from build123d import *

# Parameters (mm, degrees)
PAD_DEPTH       = 27
SKETCH001_R     = 16.5
POCKET_DEPTH    = 25
SKETCH002_R     = 16.5
POCKET001_DEPTH = 25
SKETCH003_R     = 16.5
POCKET002_DEPTH = 25
SKETCH004_R     = 16.5
POCKET003_DEPTH = 25
SKETCH005_R     = 16.5
POCKET004_DEPTH = 25
SKETCH006_R     = 16.5
POCKET005_DEPTH = 25
SKETCH007_R     = 5.125
POCKET006_DEPTH = 1.15
SKETCH008_R     = 5.125
POCKET007_DEPTH = 1.15
SKETCH009_W     = 20
SKETCH009_H     = 20
POCKET008_DEPTH = 25


with BuildPart() as part:
    # Sketch → Pad (new body)
    with BuildSketch(Plane.XY):
        with BuildLine():
            ThreePointArc((71.830952, -16.5), (78.374369, 12.374369), (49.5, 5.830952))
            ThreePointArc((49.5, 5.830952), (33, 17.5), (16.5, 5.830952))
            ThreePointArc((16.5, 5.830952), (-12.374369, 12.374369), (-5.830952, -16.5))
            ThreePointArc((-5.830952, -16.5), (-12.374369, -45.374369), (16.5, -38.830952))
            ThreePointArc((16.5, -38.830952), (33, -50.5), (49.5, -38.830952))
            ThreePointArc((49.5, -38.830952), (78.374369, -45.374369), (71.830952, -16.5))
        make_face()
        with BuildLine():
            ThreePointArc((5.830952, -16.5), (7.543698, -15.790586), (9.171788, -14.903969))
            ThreePointArc((9.171788, -14.903969), (9, -16.5), (9.171788, -18.096031))
            ThreePointArc((9.171788, -18.096031), (7.543698, -17.209414), (5.830952, -16.5))
        make_face(mode=Mode.SUBTRACT)
        with BuildLine():
            ThreePointArc((47.903969, -9.171788), (48.790586, -7.543698), (49.5, -5.830952))
            ThreePointArc((49.5, -5.830952), (50.209414, -7.543698), (51.096031, -9.171788))
            ThreePointArc((51.096031, -9.171788), (49.5, -9), (47.903969, -9.171788))
        make_face(mode=Mode.SUBTRACT)
        with BuildLine():
            ThreePointArc((18.096031, -23.828212), (17.209414, -25.456302), (16.5, -27.169048))
            ThreePointArc((16.5, -27.169048), (15.790586, -25.456302), (14.903969, -23.828212))
            ThreePointArc((14.903969, -23.828212), (16.5, -24), (18.096031, -23.828212))
        make_face(mode=Mode.SUBTRACT)
        with BuildLine():
            ThreePointArc((47.903969, -23.828212), (49.5, -24), (51.096031, -23.828212))
            ThreePointArc((51.096031, -23.828212), (50.209414, -25.456302), (49.5, -27.169048))
            ThreePointArc((49.5, -27.169048), (48.790586, -25.456302), (47.903969, -23.828212))
        make_face(mode=Mode.SUBTRACT)
        with BuildLine():
            ThreePointArc((14.903969, -9.171788), (15.790586, -7.543698), (16.5, -5.830952))
            ThreePointArc((16.5, -5.830952), (17.209414, -7.543698), (18.096031, -9.171788))
            ThreePointArc((18.096031, -9.171788), (16.5, -9), (14.903969, -9.171788))
        make_face(mode=Mode.SUBTRACT)
        with BuildLine():
            ThreePointArc((23.828212, -18.096031), (24, -16.5), (23.828212, -14.903969))
            ThreePointArc((23.828212, -14.903969), (25.456302, -15.790586), (27.169048, -16.5))
            ThreePointArc((27.169048, -16.5), (25.456302, -17.209414), (23.828212, -18.096031))
        make_face(mode=Mode.SUBTRACT)
        with BuildLine():
            ThreePointArc((42.171788, -18.096031), (40.543698, -17.209414), (38.830952, -16.5))
            ThreePointArc((38.830952, -16.5), (40.543698, -15.790586), (42.171788, -14.903969))
            ThreePointArc((42.171788, -14.903969), (42, -16.5), (42.171788, -18.096031))
        make_face(mode=Mode.SUBTRACT)
        with BuildLine():
            ThreePointArc((56.828212, -18.096031), (57, -16.5), (56.828212, -14.903969))
            ThreePointArc((56.828212, -14.903969), (58.456302, -15.790586), (60.169048, -16.5))
            ThreePointArc((60.169048, -16.5), (58.456302, -17.209414), (56.828212, -18.096031))
        make_face(mode=Mode.SUBTRACT)
    extrude(amount=PAD_DEPTH)

    # Sketch001 (on Face32 of Pad) → Pocket (cut)
    with BuildSketch(Plane.XY.offset(27)):
        Circle(SKETCH001_R)
    extrude(amount=-POCKET_DEPTH, mode=Mode.SUBTRACT)

    # Sketch002 (on Face5 of Pocket) → Pocket001 (cut)
    with BuildSketch(Plane.XY.offset(27)):
        with Locations((33, 0)):
            Circle(SKETCH002_R)
    extrude(amount=-POCKET001_DEPTH, mode=Mode.SUBTRACT)

    # Sketch003 (on Face5 of Pocket001) → Pocket002 (cut)
    with BuildSketch(Plane.XY.offset(27)):
        with Locations((66, 0)):
            Circle(SKETCH003_R)
    extrude(amount=-POCKET002_DEPTH, mode=Mode.SUBTRACT)

    # Sketch004 (on Face5 of Pocket002) → Pocket003 (cut)
    with BuildSketch(Plane.XY.offset(27)):
        with Locations((0, -33)):
            Circle(SKETCH004_R)
    extrude(amount=-POCKET003_DEPTH, mode=Mode.SUBTRACT)

    # Sketch005 (on Face5 of Pocket003) → Pocket004 (cut)
    with BuildSketch(Plane.XY.offset(27)):
        with Locations((33, -33)):
            Circle(SKETCH005_R)
    extrude(amount=-POCKET004_DEPTH, mode=Mode.SUBTRACT)

    # Sketch006 (on Face5 of Pocket004) → Pocket005 (cut)
    with BuildSketch(Plane.XY.offset(27)):
        with Locations((66, -33)):
            Circle(SKETCH006_R)
    extrude(amount=-POCKET005_DEPTH, mode=Mode.SUBTRACT)

    # Sketch007 (on Face4 of Pocket005) → Pocket006 (cut)
    with BuildSketch(Plane(origin=(0, 0, 0), x_dir=(1, 0, 0), z_dir=(0, 0, -1))):
        with Locations((16.5, 16.5)):
            Circle(SKETCH007_R)
    extrude(amount=-POCKET006_DEPTH, mode=Mode.SUBTRACT)

    # Sketch008 (on Face4 of Pocket006) → Pocket007 (cut)
    with BuildSketch(Plane(origin=(0, 0, 0), x_dir=(1, 0, 0), z_dir=(0, 0, -1))):
        with Locations((49.5, 16.5)):
            Circle(SKETCH008_R)
    extrude(amount=-POCKET007_DEPTH, mode=Mode.SUBTRACT)

    # Sketch009 (on Face43 of Pocket007) → Pocket008 (cut)
    with BuildSketch(Plane.XY.offset(27)):
        with Locations((0, 10)):
            Rectangle(SKETCH009_W, SKETCH009_H)
        with Locations((33, 10)):
            Rectangle(SKETCH009_W, SKETCH009_H)
        with Locations((66, 10)):
            Rectangle(SKETCH009_W, SKETCH009_H)
        with Locations((0, -45)):
            Rectangle(SKETCH009_W, SKETCH009_H)
        with Locations((33, -45)):
            Rectangle(SKETCH009_W, SKETCH009_H)
        with Locations((66, -45)):
            Rectangle(SKETCH009_W, SKETCH009_H)
    extrude(amount=-POCKET008_DEPTH, mode=Mode.SUBTRACT)


solid = part.part
Input: part model. Units: mm. Frame: model coordinates. A direction names the side the tool comes from. Give positions to 0.01 mm unless a question says otherwise; leave off trailing zeros. Order: outer loops, then holes, each group sorted by start corner. A loop starts at its lowest first (then second) coordinate and runs counter-clockwise, first axis right, second up. Notation, with made-up numbers: (15.25, -17) -> (53.25, -17) arc R23 cw to (53.25, 21) -> close; hole circle Ø3 at (-1, 73.25). An arc over 180 degrees is marked (long way). Use one line per item in the form item = value.
1) Mould query, pull axis Y, two halves, no side actions, for faces 4 (the cylindrical face through (58.48, -17.2, 13.31)), 5 (the flat face through (18, 8, 27)). Classes: pulls with the +Y half, pulls with the -Y half, needs draft (parallel to the pull), parting line crosses it, or undercut.
Response values:
face_4 = undercut
face_5 = needs draft
2) Line query: probe 1 along X at (y, z) = (4, 18.5); probe 2 along X at (y, z) = (-23.5, 16); probe 3 along Y at (x, z) = (77, 6.5). Output: solid intervals per line, ascending.
Response values:
probe_1 = -17.04 to -16.01, 16.01 to 16.99, 49.01 to 49.99, 82.01 to 83.04
probe_2 = -14.7 to -13.49, 13.49 to 19.51, 46.49 to 52.51, 79.49 to 80.7
probe_3 = -46.61 to -45.3, -20.7 to -19.39, -13.61 to -12.3, 12.3 to 13.61
3) Section A-A, the plane x = 25. Return loops of the section in (y, z), and give its area (3 significant figures).
Response values:
outline = (-48.56, 0) -> (-17.44, 0) -> (-17.44, 27) -> (-18.57, 27) -> (-18.57, 2) -> (-48.56, 2) -> close; (-15.56, 0) -> (15.56, 0) -> (15.56, 2) -> (-14.43, 2) -> (-14.43, 27) -> (-15.56, 27) -> close
area = 181 mm^2
4) Section B-B, the plane y = 4.5. Return loops of the section in (x, z), and give its area (3 significant figures).
Response values:
outline = (-16.91, 0) -> (82.91, 0) -> (82.91, 27) -> (81.87, 27) -> (81.87, 2) -> (50.13, 2) -> (50.13, 27) -> (48.87, 27) -> (48.87, 2) -> (17.13, 2) -> (17.13, 27) -> (15.87, 27) -> (15.87, 2) -> (-15.87, 2) -> (-15.87, 27) -> (-16.91, 27) -> close
area = 314 mm^2
5) First-contact query: pin 1 Ø16.5 at (x, y) = (37.5, -35) entering from +Z; pin 2 Ø1.4 at (y, z) = (14, 14) entering from +X; pin 3 Ø1 at (y, z) = (14, 17.5) entering from +X. Flat tips, straight axial feed; report the tip coordinate or a pass-through.
Response values:
pin_1 = 2
pin_2 = 77.37
pin_3 = 77.14
6) Section D-D, the plane x = 7.5. Return loops of the section in (y, z), and give its area (3 significant figures).
Response values:
outline = (-48.81, 0) -> (-17.19, 0) -> (-17.19, 27) -> (-18.3, 27) -> (-18.3, 2) -> (-48.81, 2) -> close; (-15.81, 0) -> (15.81, 0) -> (15.81, 2) -> (-14.7, 2) -> (-14.7, 27) -> (-15.81, 27) -> close
area = 182 mm^2
7) Reachability of faces 1 (the cylindrical face through (12.433, -13.382, 0.567)), 2 (the flat face through (-10, -14, 27)), 3 (the cylindrical face through (18.261, 7.418, 14.675)) from +Z, -Z, +X, -X, +Y, -Y: full face, straight path, thin tool, end or side. Return the list, or none.
Response values:
face_1 = -Z
face_2 = +Z, +X, -X, +Y, -Y
face_3 = +Z
